Print and shaded views of the part. All mm, measured from the part's lowest x, y and z. A direction names the side the tool comes from. Coordinates: 2 decimals unless noted, no trailing zeros. Order: outer loops, then holes, each group sorted by start corner. A loop starts at its lowest first (then second) coordinate and runs counter-clockwise, first axis right, second up.
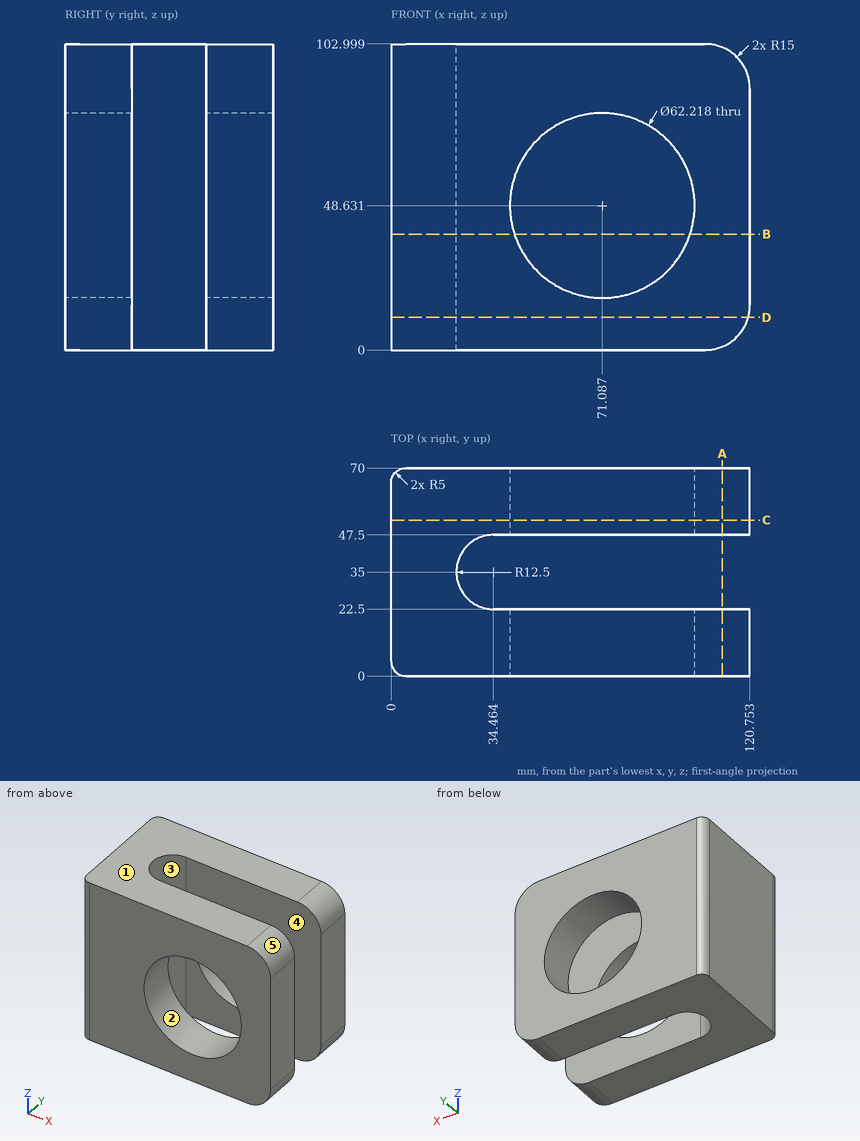
Q1. Probe line 1 (Y direction, x = 99, z = 32); line 2 (Z direction, x = 44.5, y = 4) (1 decimal); line 3 (Y direction, x = 26, z = 94). List the from-to ranges inside material, lowest first.
Established:
line 1: y = 0 to 22.5, 47.5 to 70
line 2: z = 0 to 32.5, 64.8 to 103
line 3: y = 0 to 25.8, 44.2 to 70
Q2. Which spindle directions (+Z, -Z, +X, -X, +Y, -Y) get a long thin tool onto all of the face, cutting with end or side? Do the marked faces 4 and 5. Say none if no direction does.
Established:
face 4: +Z, -Z, +X
face 5: +Z, +X, +Y, -Y
Q3. Cut at B-B, the plane z = 39. List the corners of the cut face in (x, y).
Established:
outline: (0, 5) arc R5 ccw to (5, 0) - (41.51, 0) - (41.51, 22.5) - (34.46, 22.5) arc R12.5 cw to (34.46, 47.5) - (41.51, 47.5) - (41.51, 70) - (5, 70) arc R5 ccw to (0, 65) - close; (100.67, 0) - (120.75, 0) - (120.75, 22.5) - (100.67, 22.5) - close; (100.67, 47.5) - (120.75, 47.5) - (120.75, 70) - (100.67, 70) - close
Q4. Cut at C-C, the plane y = 52.5. List the corners of the cut face in (x, z), plus the area to 3 significant figures.
Established:
outline: (0, 0) - (105.75, 0) arc R15 ccw to (120.75, 15) - (120.75, 88) arc R15 ccw to (105.75, 103) - (0, 103) - close; hole circle Ø62.22 at (71.09, 48.63)
area: 9,300 mm2
Q5. Mould opens along X. For the marked faces 1, 2 and 3 say: pulls with the +X half, pulls with the -X half, needs draft (parallel to the pull), parting line crosses it, or undercut.
Established:
face 1: needs draft
face 2: undercut
face 3: pulls with the +X half
Q6. Drop a flat-ended pin along its axis: P1, Ø10, axis at x = 97, y = 40, coming from the -Z side. Give the stop position or say it passes through.
Established:
P1: passes through
Q7. Cut at A-A, the plane x = 111.5. List the corners of the cut face in (y, z) (1 decimal), plus the area to 3 significant figures.
Established:
outline: (0, 1.1) - (22.5, 1.1) - (22.5, 101.9) - (0, 101.9) - close; (47.5, 1.1) - (70, 1.1) - (70, 101.9) - (47.5, 101.9) - close
area: 4,530 mm2
Q8. Cut at D-D, the plane z = 11. List the corners of the cut face in (x, y).
Established:
outline: (0, 5) arc R5 ccw to (5, 0) - (120.21, 0) - (120.21, 22.5) - (34.46, 22.5) arc R12.5 cw to (34.46, 47.5) - (120.21, 47.5) - (120.21, 70) - (5, 70) arc R5 ccw to (0, 65) - close
